Work out the finished part from the listing and answer in its coordinate system (mm). Face numbers are marked on the shaded views. Give positions to 0.01 mm unless a question says otherwise; leave off trailing zeros. Loops run counter-clockwise (first coordinate to the right, second up) from the corner with the lowest first, then second, coordinate; pieces in that order, holes last. Notation, with made-up numbers: (-37.5, 54) - (-23.5, 54) arc R11 cw to (-23.5, 62) - close; hole circle Ø2 at (-26.75, 80.5). An arc over 180 degrees is marked (long way). One line per item, written item: value.
from build123d import *

# Parameters (mm, degrees)
SKETCH1_R           = 150
SKETCH1_R_2         = 125
BOSS_EXTRUDE1_DEPTH = 1800
SKETCH2_R           = 160
BOSS_EXTRUDE2_DEPTH = 20
BOSS_EXTRUDE3_DEPTH = 50


with BuildPart() as part:
    # Sketch1 → Boss-Extrude1 (new body)
    with BuildSketch(Plane(origin=(0, 0, 0), x_dir=(1, 0, 0), z_dir=(0, 1, 0))):
        with Locations(Location((0, 0, 0), (0, 0, 270))):
            Circle(SKETCH1_R)
        with Locations(Location((0, 0, 0), (0, 0, 270))):
            Circle(SKETCH1_R_2, mode=Mode.SUBTRACT)
    extrude(amount=BOSS_EXTRUDE1_DEPTH)

    # Sketch2 → Boss-Extrude2 (add)
    with BuildSketch(Plane.XZ):
        with Locations(Location((0, 0, 0), (0, 0, 270))):
            Circle(SKETCH2_R)
    extrude(amount=BOSS_EXTRUDE2_DEPTH)

    # Sketch4 → Boss-Extrude3 (add, symmetric)
    with BuildSketch(Plane.XY):
        with BuildLine():
            ThreePointArc((40, -119.791280473), (0, -159.791280473), (-40, -119.791280473))
            Line((-40, -119.791280473), (-44.657114197, -114.246719929))
            ThreePointArc((-44.657114197, -114.246719929), (-2.777576385, -164.70547722), (45, -119.791280473))
            ThreePointArc((45, -119.791280473), (44.918765065, -117.088588293), (44.675353555, -114.395654025))
            Line((44.675353555, -114.395654025), (40, -119.791280473))
        make_face()
        with BuildLine():
            Line((-44.657114197, -114.246719929), (-40, -119.791280473))
            ThreePointArc((-40, -119.791280473), (0, -79.791280473), (40, -119.791280473))
            Line((40, -119.791280473), (44.675353555, -114.395654025))
            ThreePointArc((44.675353555, -114.395654025), (0.075023395, -74.791343012), (-44.657114197, -114.246719929))
        make_face()
        with BuildLine():
            Line((-123.818976335, -20), (-44.657114197, -114.246719929))
            ThreePointArc((-44.657114197, -114.246719929), (0.075023395, -74.791343012), (44.675353555, -114.395654025))
            Line((44.675353555, -114.395654025), (126.469944209, -20))
            Line((126.469944209, -20), (-123.818976335, -20))
        make_face()
    extrude(amount=BOSS_EXTRUDE3_DEPTH, both=True)


solid = part.part
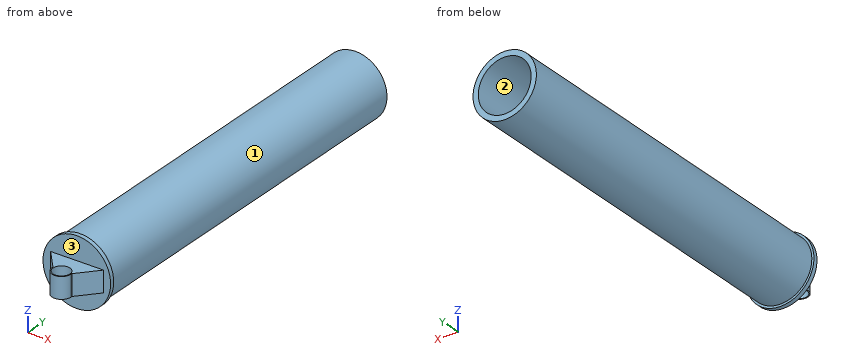
1. Section D-D (x = 74.5) is taken. Write down the section's boundary in (y, z), and give its area (3 significant figures).
Output:
outline: (-79.98, -50) - (-20, -50) - (-20, -141.6) - (0, -141.6) - (0, -130.19) - (1800, -130.19) - (1800, -100.37) - (0, -100.37) - (0, 100.37) - (1800, 100.37) - (1800, 130.19) - (0, 130.19) - (0, 141.6) - (-20, 141.6) - (-20, 50) - (-79.98, 50) - close
area: 119,000 mm²
2. Find the intervals of material crossed by line 1 along Y through (x, z) = (0, -4); line 2 along X through (y, z) = (1694, -3); line 3 along Z through (x, y) = (5, 1345), in increasing order.
Output:
line 1: y = -164.79 to -159.79, -79.79 to 0
line 2: x = -149.97 to -124.96, 124.96 to 149.97
line 3: z = -149.92 to -124.9, 124.9 to 149.92
3. Section C-C (y = 1049.5) is taken. Write down the section's boundary in (x, z).
Output:
outline: circle Ø300 at (0, 0); hole circle Ø250 at (0, 0)
4. The mould has two halves that part along Z. Classify the marked faces 1, 2 and 3: released by +Z, released by -Z, zero draft, split by the parting line, or undercut.
Output:
face 1: split by the parting line
face 2: undercut
face 3: zero draft
5. Section B-B (x = 0) is taken. Write down the section's boundary in (y, z).
Output:
outline: (-164.79, -50) - (-159.79, -50) - (-159.79, 50) - (-164.79, 50) - close; (-79.79, -50) - (-20, -50) - (-20, -160) - (0, -160) - (0, -150) - (1800, -150) - (1800, -125) - (0, -125) - (0, 125) - (1800, 125) - (1800, 150) - (0, 150) - (0, 160) - (-20, 160) - (-20, 50) - (-79.79, 50) - close
6. Flat-ended cylindrical pins translate along their axes: pin 1 Ø10 at (x, z) = (-104.5, -4.5) entering from +Y; pin 2 Ø8 at (y, z) = (1186, 36.5) entering from +X; pin 3 Ø12 at (y, z) = (465, -121) entering from +X. Find the tip coordinate at first contact, or state that the pin passes through.
Output:
pin 1: stops at y = 0
pin 2: stops at x = 146.44
pin 3: stops at x = 96.31
7. Section A-A (z = 0) is taken. Write down the section's boundary in (x, y), and give its area (3 significant figures).
Output:
outline: (-160, -20) - (-123.82, -20) - (-44.66, -114.25) arc R45 ccw (long way) to (44.68, -114.4) - (126.47, -20) - (160, -20) - (160, 0) - (150, 0) - (150, 1800) - (125, 1800) - (125, 0) - (-125, 0) - (-125, 1800) - (-150, 1800) - (-150, 0) - (-160, 0) - close; hole circle Ø80 at (0, -119.79)
area: 111,000 mm²
